Autodesk Inventor part; units mm, degrees
ref_plane "YZ Plane" through (0, 0, 0) normal (1, 0, 0) x (0, 1, 0)
ref_plane "XZ Plane" through (0, 0, 0) normal (0, 1, 0) x (-1, 0, 0)
ref_plane "XY Plane" through (0, 0, 0) normal (0, 0, 1) x (1, 0, 0)
sketch "スケッチ1" plane through (0, 0, 0) normal (0, 0, 1) x (1, 0, 0)
  line L0 (0, 3.1754) -> (2.75, 1.5877)
  line L1 (2.75, 1.5877) -> (2.75, -1.5877)
  line L2 (2.75, -1.5877) -> (0, -3.1754)
  line L3 (0, -3.1754) -> (-2.75, -1.5877)
  line L4 (-2.75, -1.5877) -> (-2.75, 1.5877)
  line L5 (-2.75, 1.5877) -> (0, 3.1754)
  point P0 (0, 0)
  point P1 (0, 0)
  dimension "d0" = 5.5
extrude "押し出し1" add sketch "スケッチ1" along normal blind 12
sketch "スケッチ2" plane through (0, 0, 12) normal (0, 0, 1) x (1, 0, 0)
  circle A0 centre (0, 0) radius 1.5
  dimension "d3" = 3
extrude "押し出し2" add sketch "スケッチ2" along normal blind 5
thread "ねじ1"
chamfer "面取り1" distance 0.3 angle 45 1 edges at (-1.5, 0, 17)
fillet "フィレット1" radius 0.1 18 edges at (-1.375, 2.3816, 12) (1.375, 2.3816, 12) (2.75, 0, 12) (1.375, -2.3816, 12) (-1.375, -2.3816, 12) (-2.75, 0, 12) (-2.75, -1.5877, 6) (0, -3.1754, 6) (2.75, -1.5877, 6) (2.75, 1.5877, 6) (0, 3.1754, 6) (-2.75, 1.5877, 6) (-1.375, 2.3816, 0) (1.375, 2.3816, 0) (2.75, 0, 0) (1.375, -2.3816, 0) (-1.375, -2.3816, 0) (-2.75, 0, 0)
sketch "スケッチ3" plane through (0, 0, 0) normal (0, 0, -1) x (-1, 0, 0)
  point P0 (0, 0)
hole "穴1" at (0, 0, 0) direction (0, 0, 1) diameter 2.459 depth 5 tip angle 118
chamfer "面取り2" distance 0.2 angle 45 1 edges at (0, -1.2295, 0)
properties part number "hexagonal_spacer_M3_12mm" material "ABS プラスチック"
Input: part model. Units: mm. Frame: model coordinates. A direction names the side the tool comes from. Coordinates: 2 decimals unless noted, no trailing zeros. Order: outer loops, then holes, each group sorted by start corner. A loop starts at its lowest first (then second) coordinate and runs counter-clockwise, first axis right, second up.
1. Ray query, line 1 along X through (y, z) = (0, 2.45); line 2 along Y through (x, z) = (0, 2.45); line 3 along Z through (x, y) = (2, 1.75). Return the intervals inside material, ascending.
Checked values:
line 1: x = -2.75 to -1.23, 1.23 to 2.75
line 2: y = -3.16 to -1.23, 1.23 to 3.16
line 3: z = 0 to 12
2. Cut plane B-B, the plane z = 10.5. Return loops of the section in (x, y).
Checked values:
outline: (-2.75, -1.53) arc R0.1 ccw to (-2.7, -1.62) - (-0.05, -3.15) arc R0.1 ccw to (0.05, -3.15) - (2.7, -1.62) arc R0.1 ccw to (2.75, -1.53) - (2.75, 1.53) arc R0.1 ccw to (2.7, 1.62) - (0.05, 3.15) arc R0.1 ccw to (-0.05, 3.15) - (-2.7, 1.62) arc R0.1 ccw to (-2.75, 1.53) - close
3. Draft query along X for faces 1 (the conical face through (0.064, 0.204, 5.61)), 2 (the flat face through (-1.2, -1.3, 0)), 3 (the flat face through (-2.75, 0, 6)). Return one class per face: +X half, -X half, draft (parallel to the pull), parting line (faces both ways), or undercut.
Checked values:
face 1: undercut
face 2: draft
face 3: -X half
4. Cut plane C-C, the plane z = 15. Return loops of the section in (x, y).
Checked values:
outline: circle Ø3 at (0, 0)
5. Access query for faces 4 (the flat face through (1.1, -1.3, 12)), 5 (the flat face through (-1.394, 2.371, 5.917)), 6 (the cylindrical face through (0.748, -0.976, 2.634)). Directions: +Z, -Z, +X, -X, +Y, -Y. A direction counts if a zero-diameter tool reaches every point of the face in a straight line with its end or side. Return the directions, or none.
Checked values:
face 4: +Z
face 5: +Z, -Z, -X, +Y
face 6: -Z
6. Contact query for flat-ended pins moving along their axis: P1, Ø2.5, axis at x = 0.5, y = -1.5, coming from the +Z side; P2, Ø3, axis at y = 1.5, z = 14, coming from the -X side; P3, Ø1.5, axis at x = 0, y = 0, coming from the -Z side. Output: stop coordinate, or through.
Checked values:
P1: stops at z = 17
P2: stops at x = -1.5
P3: stops at z = 5.29
7. Cut plane A-A, the plane z = 1.75. Return loops of the section in (x, y).
Checked values:
outline: (-2.75, -1.53) arc R0.1 ccw to (-2.7, -1.62) - (-0.05, -3.15) arc R0.1 ccw to (0.05, -3.15) - (2.7, -1.62) arc R0.1 ccw to (2.75, -1.53) - (2.75, 1.53) arc R0.1 ccw to (2.7, 1.62) - (0.05, 3.15) arc R0.1 ccw to (-0.05, 3.15) - (-2.7, 1.62) arc R0.1 ccw to (-2.75, 1.53) - close; hole circle Ø2.46 at (0, 0)
